Part model, mm, in its own coordinate system. A direction names the side the tool comes from. Give positions to 0.01 mm unless a question says otherwise; leave off trailing zeros. Order: outer loops, then holes, each group sorted by start corner. A loop starts at its lowest first (then second) coordinate and runs counter-clockwise, first axis right, second up. Notation, with made-up numbers: (45, 25.5) - (78, 25.5) arc R18 cw to (78, 46.5) - close; hole circle Ø10 at (-29.75, -37.5). An arc over 180 degrees is marked (long way). Use one line per item in the form item = value. Start each with the question number.
1. Drill centre lines: line 1 (Y direction, x = 2.1, z = -7.5) (1 decimal); line 2 (Z direction, x = 4.55, y = 11); line 3 (Y direction, x = 3.35, z = -18.5) (3 decimals). Where is each one in solid material? Low to high.
2. Band-saw the part on D-D, the plane z = -20. List the corners of the cut face in (x, y) (1 decimal), plus the area to 3 significant figures.
3. Band-saw the part on A-A, the plane z = -6. List the corners of the cut face in (x, y) (1 decimal), plus the area to 3 significant figures.
4. Tool access for faces 4 (the face through (3.197, 14.331, -12.365)), 5 (the face through (2, 11, 0)), 6 (the face through (2, 11, -9.462)): list every direction of +Z, -Z, +X, -X, +Y, -Y with a clear straight run to the whole face (end or side of a thin tool).
5. Pull direction Y, two halves, no side cores. Call faces 1 (the face through (2, 0, -16)), 2 (the face through (2, 17.59, -25)), 3 (the face through (2, 11, -31.75)): +Y half, -Y half, draft (parallel to the pull), parting line (faces both ways), or undercut.
6. Band-saw the part on B-B, the plane x = 4. State how many separate pieces and enclosed holes the cut face has, plus the area to 3 significant figures.
7. Pin check, flat tip, straight feed: P1, Ø5, axis at y = 11.11, z = -15.88, coming from the +X side. Stop position of the tip, or through.
Autodesk Inventor part; units mm, degrees
ref_plane "YZ Plane" through (0, 0, 0) normal (1, 0, 0) x (0, 1, 0)
ref_plane "XZ Plane" through (0, 0, 0) normal (0, 1, 0) x (-1, 0, 0)
ref_plane "XY Plane" through (0, 0, 0) normal (0, 0, 1) x (1, 0, 0)
sketch "Sketch1" plane through (0, 0, 0) normal (1, 0, 0) x (0, 1, 0)
  line L0 (22.225, 0) -> (22.225, -31.75)
  line L1 (22.225, -31.75) -> (0, -31.75)
  line L2 (0, -31.75) -> (0, 0)
  line L3 (17.5895, -4.446) -> (4.5769, -4.446)
  line L4 (6.35, -31.75) -> (25.4, -31.75)
  line L5 (0, 0) -> (4.7625, 0)
  line L6 (17.5895, 0) -> (22.225, 0)
  line L7 (4.6355, -22.225) -> (17.5895, -22.225)
  line L8 (17.5895, -22.225) -> (17.5895, -27.2415)
  line L9 (17.5895, -27.2415) -> (4.6355, -27.2415)
  line L10 (4.6355, -27.2415) -> (4.6355, -22.225)
  line L11 (22.225, 0) -> (0, 0)
  line L12 (17.5895, -4.446) -> (4.6355, -4.446)
  line L13 (4.6355, -4.446) -> (4.6355, -9.4625)
  line L14 (4.6355, -9.4625) -> (17.5895, -9.4625)
  line L15 (17.5895, -9.4625) -> (17.5895, -4.446)
  dimension "d8" = 12.954
  dimension "d9" = 5.0165
  dimension "d10" = 4.5085
  dimension "d11" = 4.6355
  dimension "d28" = 4.6355
  dimension "d37" = 31.75
  dimension "d38" = 31.75
  dimension "d43" = 5.0165
  dimension "d48" = 12.954
  dimension "d49" = 4.6355
extrude "Extrusion1" add sketch "Sketch1" along normal blind 4.7625 contours L0 L1 L2 L5 L11 L6 | L15 L14 L13 L3
sketch "Sketch2" plane through (4.7625, 0, 0) normal (1, 0, 0) x (0, 0, -1)
  line L0 (22.225, 17.5895) -> (27.2415, 17.5895)
  line L1 (27.2415, 17.5895) -> (27.2415, 4.6355)
  line L2 (27.2415, 4.6355) -> (22.225, 4.6355)
  line L3 (22.225, 4.6355) -> (22.225, 17.5895)
  line L4 (0, 0) -> (31.75, 0)
  line L5 (31.75, 0) -> (31.75, 22.225)
  line L6 (31.75, 22.225) -> (0, 22.225)
  circle A0 centre (15.875, 11.1125) radius 4.7625
  line L7 (0, 22.225) -> (0, 0)
  dimension "d14" = 9.525
  dimension "d15" = 11.1125
  dimension "d39" = 22.225
  dimension "d52" = 31.75
  dimension "d53" = 15.875
extrude "Extrusion2" cut sketch "Sketch2" against normal blind 3.175 contours A0
extrude "Extrusion5" cut sketch "Sketch1" along normal blind 25.4 contours L15 L14 L13 L3
sketch "Sketch5" plane through (4.7625, 0, 0) normal (1, 0, 0) x (0, 0, -1)
  circle A0 centre (15.875, 11.1125) radius 4.7625
  point P0 (0, 0)
hole "Hole1" at (4.7625, 11.1125, -15.875) direction (-1, 0, 0) diameter 3.683 depth 14.9352 tip angle 118
fillet "Fillet1" radius 0.381 26 edges at (0, 22.225, -15.875) (2.3813, 22.225, 0) (4.7625, 22.225, -15.875) (4.7625, 11.1125, -31.75) (0, 11.1125, -31.75) (4.7625, 0, -15.875) (2.3813, 0, -31.75) (4.7625, 11.1125, 0) (4.7625, 11.1125, -4.446) (4.7625, 17.5895, -6.9542) (4.7625, 11.1125, -9.4625) (4.7625, 4.6355, -6.9542) (0, 4.6355, -6.9542) (0, 11.1125, -4.446) (2.3813, 22.225, -31.75) (4.7625, 17.5895, -24.7332) (4.7625, 11.1125, -22.225) (4.7625, 4.6355, -24.7332) (4.7625, 11.1125, -27.2415) (0, 17.5895, -24.7332) (0, 11.1125, -27.2415) (0, 11.1125, -22.225) (0, 4.6355, -24.7332) (0, 11.1125, -9.4625) (0, 17.5895, -6.9542) (0, 0, -15.875)
equation "\"d28\" = d11"
equation "\"d38\" = d37"
equation "\"d15\" = 0.5 * d39"
equation "\"d53\" = 0.5 * d52"
equation "\"d32\" = 0.5 * d31"
properties part number "TensionerPlate"
From the geometry:
q1.line_1 = 0 to 4.6, 17.6 to 22.2
q1.line_2 = -31.71 to -27.28, -22.19 to -20.64, -11.11 to -9.5, -4.41 to -0.04
q1.line_3 = 0 to 7.139, 15.086 to 22.225
q2.outline = (0, 0.4) arc R0.4 ccw to (0.4, 0) - (4.4, 0) arc R0.4 ccw to (4.8, 0.4) - (4.8, 8.7) - (1.6, 8.7) - (1.6, 13.5) - (4.8, 13.5) - (4.8, 21.8) arc R0.4 ccw to (4.4, 22.2) - (0.4, 22.2) arc R0.4 ccw to (0, 21.8) - close
q2.area = 90.6 mm²
q3.outline = (0, 0.4) arc R0.4 ccw to (0.4, 0) - (4.4, 0) arc R0.4 ccw to (4.8, 0.4) - (4.8, 4.3) arc R0.4 ccw to (4.4, 4.6) - (0.4, 4.6) arc R0.4 ccw to (0, 4.3) - close; (0, 18) arc R0.4 ccw to (0.4, 17.6) - (4.4, 17.6) arc R0.4 ccw to (4.8, 18) - (4.8, 21.8) arc R0.4 ccw to (4.4, 22.2) - (0.4, 22.2) arc R0.4 ccw to (0, 21.8) - close
q3.area = 43.9 mm²
q4.face_4 = +X
q4.face_5 = +Z, +X, -X, +Y, -Y
q4.face_6 = +X, -X
q5.face_1 = -Y half
q5.face_2 = undercut
q5.face_3 = draft
q6.separate_pieces = 1
q6.enclosed_holes = 3
q6.area = 504 mm²
q7.P1 = 1.59
